```python
from build123d import *

# Parameters (mm, degrees)
SKETCH5_W                       = 20.209666631
SKETCH5_H                       = 20.346218433
BOSS_EXTRUDE3_DEPTH             = 20.32
DRAFT4_ANGLE                    = 4
DRAFT5_ANGLE                    = 4
SKETCH6_W                       = 10.134168445
SKETCH6_H                       = 17.341048708
BOSS_EXTRUDE4_DEPTH             = 20.32
SKETCH7_W                       = 6.151087315
SKETCH7_H                       = 12.30217463
BOSS_EXTRUDE5_DEPTH             = 20.32
CUT_EXTRUDE1_DEPTH              = 20.32
SKETCH9_W                       = 6.151087315
SKETCH9_H                       = 16.039002112
BOSS_EXTRUDE8_DEPTH             = 12.7
F_0_80_TAPPED_HOLE1_D           = 1.19126
F_0_80_TAPPED_HOLE1_DEPTH       = 4.0005
F_0_80_TAPPED_HOLE1_CSINK_D     = 3.0226
F_0_80_TAPPED_HOLE1_CSINK_ANGLE = 100
F_0_80_TAPPED_HOLE1_TIP         = 0.357890611
F_0_80_TAPPED_HOLE3_D           = 1.19126
F_0_80_TAPPED_HOLE3_DEPTH       = 4.064
F_0_80_TAPPED_HOLE3_CSINK_D     = 3.0226
F_0_80_TAPPED_HOLE3_CSINK_ANGLE = 100
F_0_80_TAPPED_HOLE3_TIP         = 0.357890611
SKETCH28_W                      = 35.682781241
SKETCH28_H                      = 76.087494434
BOSS_EXTRUDE13_DEPTH            = 11.938
FILLET5_R                       = 6.35
FILLET6_R                       = 6.35


with BuildPart() as part:
    # Sketch5 → Boss-Extrude3 (new body)
    with BuildSketch(Plane.XY):
        with Locations((-110.129027961, 66.022796056)):
            Rectangle(SKETCH5_W, SKETCH5_H)
    extrude(amount=BOSS_EXTRUDE3_DEPTH)

    # Draft4
    draft4_faces = [part.faces().sort_by_distance(p)[0] for p in [
        (-100.024194645, 66.022796056, 10.16),
        (-120.233861276, 66.022796056, 10.16),
        (-110.129027961, 66.022796056, 20.32),
    ]]
    draft(draft4_faces, Plane(origin=(-120.233861276, 55.849686839, 20.32), x_dir=(0, 0, -1), z_dir=(0, -1, 0)), DRAFT4_ANGLE)

    # Draft5
    draft5_faces = [part.faces().sort_by_distance(p)[0] for p in [
        (-110.129027961, 66.245821761, 0),
    ]]
    draft(draft5_faces, Plane(origin=(-120.233861276, 55.849686839, 20.32), x_dir=(0, 0, -1), z_dir=(0, -1, 0)), DRAFT5_ANGLE)

    # Sketch6 → Boss-Extrude4 (add)
    with BuildSketch(Plane.XY):
        with Locations((-110.017330359, 47.179162485)):
            Rectangle(SKETCH6_W, SKETCH6_H)
    extrude(amount=BOSS_EXTRUDE4_DEPTH)

    # Sketch7 → Boss-Extrude5 (add)
    with BuildSketch(Plane.XY):
        with Locations((-110.013841195, 32.357550816)):
            Rectangle(SKETCH7_W, SKETCH7_H)
    extrude(amount=BOSS_EXTRUDE5_DEPTH)

    # Sketch8 → Cut-Extrude1 (cut)
    with BuildSketch(Plane(origin=(0, 0, 0), x_dir=(-1, 0, 0), z_dir=(0, 0, -1))):
        Polygon((113.089384852, 38.508638131), (113.089384852, 41.703281679), (106.938297537, 41.703281679), (106.938297537, 38.508638131), (106.938297537, 26.206463501), (113.089384852, 26.206463501), align=None)
    extrude(amount=-CUT_EXTRUDE1_DEPTH, mode=Mode.SUBTRACT)

    # Sketch9 → Boss-Extrude8 (add)
    with BuildSketch(Plane.XZ.offset(-41.703281679)):
        with Locations((-110.013841195, 10.15769714)):
            Rectangle(SKETCH9_W, SKETCH9_H)
    extrude(amount=BOSS_EXTRUDE8_DEPTH)

    # #0-80 Tapped Hole1
    with Locations(Plane(origin=(-104.950246136, 0, 0), x_dir=(0, 0, -1), z_dir=(1, 0, 0))):
        with Locations((-10.606199537, 40.03468966)):
            CounterSinkHole(F_0_80_TAPPED_HOLE1_D / 2, F_0_80_TAPPED_HOLE1_CSINK_D / 2, depth=F_0_80_TAPPED_HOLE1_DEPTH, counter_sink_angle=F_0_80_TAPPED_HOLE1_CSINK_ANGLE)
            with Locations((0, 0, -(F_0_80_TAPPED_HOLE1_DEPTH + F_0_80_TAPPED_HOLE1_TIP / 2))):  # 118° drill point
                Cone(0, F_0_80_TAPPED_HOLE1_D / 2, F_0_80_TAPPED_HOLE1_TIP, mode=Mode.SUBTRACT)

    # #0-80 Tapped Hole3
    with Locations(Plane.ZY.offset(115.084414581)):
        with Locations((10.610590501, 40.003135548)):
            CounterSinkHole(F_0_80_TAPPED_HOLE3_D / 2, F_0_80_TAPPED_HOLE3_CSINK_D / 2, depth=F_0_80_TAPPED_HOLE3_DEPTH, counter_sink_angle=F_0_80_TAPPED_HOLE3_CSINK_ANGLE)
            with Locations((0, 0, -(F_0_80_TAPPED_HOLE3_DEPTH + F_0_80_TAPPED_HOLE3_TIP / 2))):  # 118° drill point
                Cone(0, F_0_80_TAPPED_HOLE3_D / 2, F_0_80_TAPPED_HOLE3_TIP, mode=Mode.SUBTRACT)

    # Sketch28 → Boss-Extrude13 (add)
    with BuildSketch(Plane(origin=(0, 29.003281679, 0), x_dir=(-1, 0, 0), z_dir=(0, -1, 0))):
        with Locations((109.89388319, -12.810019293)):
            Rectangle(SKETCH28_W, SKETCH28_H)
    extrude(amount=BOSS_EXTRUDE13_DEPTH)

    # Fillet5
    # the kernel refuses this fillet: 6.35 mm, written as the material it takes off along each edge
    with BuildSketch(Plane(origin=(-76.177492569, 17.065281679, -25.233727924), x_dir=(0, 1, 0), z_dir=(-1, 0, 0))) as fillet5_piece_1:
        with BuildLine():
            CenterArc((FILLET5_R, -FILLET5_R), FILLET5_R, 90, 90)
            Line((0, -FILLET5_R), (0, 0))
            Line((0, 0), (FILLET5_R, 0))
        make_face()
    extrude(amount=67.43278124, mode=Mode.SUBTRACT)
    with BuildSketch(Plane(origin=(-76.177492569, 29.003281679, -25.233727924), x_dir=(0, -1, 0), z_dir=(-1, 0, 0))) as fillet5_piece_2:
        with BuildLine():
            CenterArc((FILLET5_R, FILLET5_R), FILLET5_R, 180, 90)
            Line((0, FILLET5_R), (0, 0))
            Line((0, 0), (FILLET5_R, 0))
        make_face()
    extrude(amount=67.43278124, mode=Mode.SUBTRACT)

    # Fillet6
    # the kernel refuses this fillet: 6.35 mm, written as the material it takes off along each edge
    with BuildSketch(Plane(origin=(-143.61027381, 17.065281679, 50.85376651), x_dir=(0, 1, 0), z_dir=(1, 0, 0)), Plane(origin=(-143.61027381, 29.003281679, 50.85376651), x_dir=(0, 0, -1), z_dir=(1, 0, 0))) as fillet6_piece_1:
        with BuildLine():
            CenterArc((FILLET6_R, -FILLET6_R), FILLET6_R, 90, 90)
            Line((0, -FILLET6_R), (0, 0))
            Line((0, 0), (FILLET6_R, 0))
        make_face()
    extrude(amount=67.43278124, mode=Mode.SUBTRACT)


solid = part.part
```
Can you work these out from the model? Positions are in its coordinate system, mm. A direction names the side the tool comes from. Round coordinates to 2 decimals unless told otherwise and drop trailing zeros. Loops run counter-clockwise (first coordinate to the right, second up) from the corner with the lowest first, then second, coordinate; pieces in that order, holes last. Notation, with made-up numbers: M 54,2.25 L 97,2.25 A24 cw 97,40.25 Z; hole C 24,11.5 d6. An arc over 180 degrees is marked long. Answer as a JSON object with one key per item and string values. Group by question number.
Q1. Imagine slicing it at A-A, the plane x = -101.5. Please give me the cut outline in (y, z), then the cut area to 3 significant figures.
Q2. Will these pins go through, and if not, where does the flat tip stop? pin 1 (10 mm diameter, centred on x = -102, y = 30, fed in from -Z); pin 2 (8 mm diameter, centred on y = 36, z = -1.5, fed in from +X); pin 3 (19 mm diameter, centred on y = 46.5, z = 14, fed in from -X).
Q3. On a 3-axis mill with a long thin cutter (end or side, diameter ignored), from which of +Z, -Z, +X, -X, +Y, -Y can I reach the whole of each face in a straight line? I mean faces 1 (the flat face through (-106.938, 40, 19)), 2 (the flat face through (-110, 47, 0)), 3 (the flat face through (-110.29, 66.17, 21.04)), 4 (the flat face through (-104.95, 47, 10)). Say none if no direction works.
Q4. Imagine slicing it at C-C, the plane y = 53.5. Please give me the cut outline in (x, z), then the cut area to 3 significant figures.
Q5. Imagine slicing it at D-D, the plane x = -124. Please give me the cut outline in (y, z).
Q6. We'd pull the mould along Y, two halves only. Please class faces 5 (the flat face through (-92.052, 23, 13)), 6 (the cylindrical face through (-109.64, 27.32, -23.19)), 7 (the flat face through (-106.938, 40, 1)), 8 (the flat face through (-110, 17.065, 12)): +Y half, -Y half, draft (parallel to the pull), parting line (faces both ways), or undercut.
Q7. Imagine slicing it at B-B, the plane z = 4. Please give me the cut outline in (x, y), then the cut area to 3 significant figures.
Q8. Please list where these lines run through material, in increasing order: L1, parallel to Y at x = -123, z = 15.5; L2, parallel to Y at x = -106, z = 1; L3, parallel to Z at x = -112, y = 31.5.
Findings:
{
 "1": {"outline": "M 17.07,-18.88 A6.35 ccw 23.03,-25.22 A6.35 ccw 29,-18.88 L 29,44.5 A6.35 ccw 23.03,50.84 A6.35 ccw 17.07,44.5 Z; M 55.85,0 L 76.2,-1.42 L 76.2,21.74 L 55.85,20.32 Z", "area": "1,320 mm2"},
 "2": {"pin 1": "stops at z = -24.78", "pin 2": "stops at x = -104.95", "pin 3": "stops at x = -120.24"},
 "3": {"face 1": "+Z", "face 2": "-Z, +X, -X", "face 3": "+Z, +X, -X", "face 4": "+Z, -Z, +X"},
 "4": {"outline": "M -115.08,0 L -104.95,0 L -104.95,20.32 L -115.08,20.32 Z", "area": "206 mm2"},
 "5": {"outline": "M 17.07,-18.88 A6.35 ccw 23.03,-25.22 A6.35 ccw 29,-18.88 L 29,44.5 A6.35 ccw 23.03,50.84 A6.35 ccw 17.07,44.5 Z"},
 "6": {"face 5": "draft", "face 6": "+Y half", "face 7": "undercut", "face 8": "-Y half"},
 "7": {"outline": "M -127.74,17.07 L -92.05,17.07 L -92.05,29 L -106.94,29 L -106.94,38.51 L -104.95,38.51 L -104.95,55.85 L -100.02,55.85 L -98.6,76.2 L -121.66,76.2 L -120.23,55.85 L -115.08,55.85 L -115.08,38.51 L -113.09,38.51 L -113.09,29 L -127.74,29 Z", "area": "1,100 mm2"},
 "8": {"L1": "y = 17.07 to 29", "L2": "y = 17.07 to 29, 38.51 to 76.2", "L3": "z = 2.14 to 18.18"}
}
